```python
from build123d import *

# Parameters (mm, degrees)
CROQUIS1_R              = 12.5
CROQUIS1_R_2            = 3
SALIENTE_EXTRUIR1_DEPTH = 3
REDONDEO1_R             = 0.5


with BuildPart() as part:
    # Croquis1 → Saliente-Extruir1 (new body)
    with BuildSketch(Plane(origin=(0, 0, 0), x_dir=(1, 0, 0), z_dir=(0, 1, 0))):
        with Locations(Location((0, 0, 0), (0, 0, 270))):
            Circle(CROQUIS1_R)
        with Locations(Location((0, 0, 0), (0, 0, 270))):
            Circle(CROQUIS1_R_2, mode=Mode.SUBTRACT)
    extrude(amount=SALIENTE_EXTRUIR1_DEPTH)

    # Redondeo1
    redondeo1_edges = [part.edges().sort_by_distance(p)[0] for p in [
        (0, 0, -12.5),
        (0, 3, -12.5),
        (0, 0, -3),
        (0, 3, -3),
    ]]
    fillet(redondeo1_edges, radius=REDONDEO1_R)


solid = part.part
```
Source: CAD feature listing. Evaluate the final solid. Frame: model axes, mm. Round coordinates to 2 decimals unless told otherwise and drop trailing zeros. Write each loop counter-clockwise with the first axis right and the second up, starting at its lowest first coordinate (ties: lowest second). Pieces come first, ordered by that corner, then holes. Notation, with made-up numbers: M -18,41 L 22,41 A16 cw 22,48 Z; hole C 83.5,77.5 d1. An arc over 180 degrees is marked long. Use CSV: the item, a comma, the result in double quotes. Start each with the question number.
Q1. Cut plane A-A on x = 0. Output: boundary loops of the cut face in (y, z).
Q2. First-contact query: P1, Ø1.5, axis at x = 4.5, y = 2, coming from the +Z side. Flat tip, straight axial feed; report the tip coordinate or a pass-through.
Q3. Cut plane C-C on y = 1.05. Output: boundary loops of the cut face in (x, z), plus the area to 3 significant figures.
Q4. Pull-direction query (Z, two-part tool) for faces 1 (the face through (3.755, 1.486, 11.923)), 2 (the face through (0.9, 1.49, 2.86)), 3 (the face through (2.8, 3, 2.5)); classes: +Z half, -Z half, draft (parallel to the pull), parting line (faces both ways), or undercut.
Q5. Cut plane B-B on z = 0. Output: boundary loops of the cut face in (x, y), plus the area to 3 significant figures.
Q6. Line query: line 1 (X direction, y = 1.2, z = 0); line 2 (Z direction, x = -2, y = 1.1); line 3 (Z direction, x = 2.25, y = 0.75). Output: solid intervals per line, ascending. Write a range as from..to.
Results found:
1,outline,"M 0,-12 A0.5 ccw 0.5,-12.5 L 2.5,-12.5 A0.5 ccw 3,-12 L 3,-3.5 A0.5 ccw 2.5,-3 L 0.5,-3 A0.5 ccw 0,-3.5 Z; M 0,3.5 A0.5 ccw 0.5,3 L 2.5,3 A0.5 ccw 3,3.5 L 3,12 A0.5 ccw 2.5,12.5 L 0.5,12.5 A0.5 ccw 0,12 Z"
2,P1,"z = 11.92"
3,outline,"C 0,0 d25; hole C 0,0 d6"
3,area,"463 mm^2"
4,face 1,"parting line"
4,face 2,"undercut"
4,face 3,"draft"
5,outline,"M -12.5,0.5 A0.5 ccw -12,0 L -3.5,0 A0.5 ccw -3,0.5 L -3,2.5 A0.5 ccw -3.5,3 L -12,3 A0.5 ccw -12.5,2.5 Z; M 3,0.5 A0.5 ccw 3.5,0 L 12,0 A0.5 ccw 12.5,0.5 L 12.5,2.5 A0.5 ccw 12,3 L 3.5,3 A0.5 ccw 3,2.5 Z"
5,area,"56.6 mm^2"
6,line 1,"-12.5..-3, 3..12.5"
6,line 2,"-12.34..-2.24, 2.24..12.34"
6,line 3,"-12.3..-1.98, 1.98..12.3"
